```python
from build123d import *

# Parameters (mm, degrees)
F1_DEPTH = 36
F2_R     = 2.2
F3_DEPTH = 3.001


with BuildPart() as f1:
    # F0 (on Front) → F1 (new body)
    with BuildSketch(Plane.XZ):
        Polygon((-36, 0), (0, 0), (27.5776, 23.140354), (26.033813, 25.761185), (-1.091911, 3), (-36, 3), align=None)
    extrude(amount=F1_DEPTH)

    # F2 (on face) → F3 (cut, through all)
    with BuildSketch(Plane.XY.offset(3)):
        with Locations((-30, -9)):
            Circle(F2_R)
        with Locations((-30, -27)):
            Circle(F2_R)
    extrude(amount=-F3_DEPTH, mode=Mode.SUBTRACT)


solid = f1.part
```
Input: part model. Units: mm. Frame: model coordinates. Round coordinates to 2 decimals unless told otherwise and drop trailing zeros. Loops run counter-clockwise (first coordinate to the right, second up) from the corner with the lowest first, then second, coordinate; pieces in that order, holes last.
1) Section query D-D on y = -3. Return the cut outline in (x, z).
Ans:
outline: (-36, 0) - (0, 0) - (27.58, 23.14) - (26.03, 25.76) - (-1.09, 3) - (-36, 3) - close
2) Pull-direction query (X, two-part tool) for faces 1 (the flat face through (13.6, -17.75, 11.41)), 2 (the cylindrical face through (-30.477, -29.148, 1.521)), 3 (the flat face through (-18, -18, 3)), 4 (the cylindrical face through (-31.62, -7.51, 1.52)); classes: released by +X, released by -X, zero draft, split by the parting line, or undercut.
Ans:
face 1: released by +X
face 2: undercut
face 3: zero draft
face 4: undercut
3) Pin query (flat end, axial travel): pin 1 (7 mm diameter, centred on x = -30, y = -9, fed in from +Z); pin 2 (8 mm diameter, centred on y = -13, z = 17, fed in from +X); pin 3 (1.5 mm diameter, centred on y = -18.5, z = 20.5, fed in from +X). Return the tip coordinate at first contact, or that it passes through.
Ans:
pin 1: stops at z = 3
pin 2: stops at x = 25.03
pin 3: stops at x = 25.32
4) Section query A-A on y = -27. Return the cut outline in (x, z).
Ans:
outline: (-36, 0) - (-32.2, 0) - (-32.2, 3) - (-36, 3) - close; (-27.8, 0) - (0, 0) - (27.58, 23.14) - (26.03, 25.76) - (-1.09, 3) - (-27.8, 3) - close
5) Section query B-B on x = -30. Return the cut outline in (y, z).
Ans:
outline: (-36, 0) - (-29.2, 0) - (-29.2, 3) - (-36, 3) - close; (-24.8, 0) - (-11.2, 0) - (-11.2, 3) - (-24.8, 3) - close; (-6.8, 0) - (0, 0) - (0, 3) - (-6.8, 3) - close
6) Section query C-C on x = -12. Return the cut outline in (y, z), plus the area to 3 significant figures.
Ans:
outline: (-36, 0) - (0, 0) - (0, 3) - (-36, 3) - close
area: 108 mm2
7) Material intervals for line 1 (Y direction, x = -30, z = 1.35); line 2 (Z direction, x = -7.5, y = -13); line 3 (X direction, y = -11, z = 2.75), sorted ascending.
Ans:
line 1: y = -36 to -29.2, -24.8 to -11.2, -6.8 to 0
line 2: z = 0 to 3
line 3: x = -36 to -30.92, -29.08 to 3.28
